```python
from build123d import *

# Parameters (mm, degrees)
SKETCH_1_R      = 63
SKETCH_1_R_2    = 1.25
EXTRUDE_1_DEPTH = 15
FILLET_1_R      = 3


with BuildPart() as part:
    # 草图1 → 凸台-拉伸1 (new body)
    with BuildSketch(Plane.XY):
        Circle(SKETCH_1_R)
        with Locations((0, 55)):
            Circle(SKETCH_1_R_2, mode=Mode.SUBTRACT)
        with Locations((47.631397208, 27.5)):
            Circle(SKETCH_1_R_2, mode=Mode.SUBTRACT)
        with Locations((47.631397208, -27.5)):
            Circle(SKETCH_1_R_2, mode=Mode.SUBTRACT)
        with Locations((0, -55)):
            Circle(SKETCH_1_R_2, mode=Mode.SUBTRACT)
        with Locations((-47.631397208, -27.5)):
            Circle(SKETCH_1_R_2, mode=Mode.SUBTRACT)
        with Locations((-47.631397208, 27.5)):
            Circle(SKETCH_1_R_2, mode=Mode.SUBTRACT)
        with BuildLine():
            Line((-2.5, 55), (-2.724459655, 59.938112413))
            ThreePointArc((-2.724459655, 59.938112413), (-30, 51.961524227), (-50.545698177, 32.328507479))
            Line((-50.545698177, 32.328507479), (-46.381397208, 29.665063509))
            ThreePointArc((-46.381397208, 29.665063509), (-45.466333699, 26.25), (-48.881397208, 25.334936491))
            Line((-48.881397208, 25.334936491), (-53.270157832, 27.609604933))
            ThreePointArc((-53.270157832, 27.609604933), (-60, 0), (-53.270157832, -27.609604933))
            Line((-53.270157832, -27.609604933), (-48.881397208, -25.334936491))
            ThreePointArc((-48.881397208, -25.334936491), (-45.466333699, -26.25), (-46.381397208, -29.665063509))
            Line((-46.381397208, -29.665063509), (-50.545698177, -32.328507479))
            ThreePointArc((-50.545698177, -32.328507479), (-30, -51.961524227), (-2.724459655, -59.938112413))
            Line((-2.724459655, -59.938112413), (-2.5, -55))
            ThreePointArc((-2.5, -55), (0, -52.5), (2.5, -55))
            Line((2.5, -55), (2.724459655, -59.938112413))
            ThreePointArc((2.724459655, -59.938112413), (30, -51.961524227), (50.545698177, -32.328507479))
            Line((50.545698177, -32.328507479), (46.381397208, -29.665063509))
            ThreePointArc((46.381397208, -29.665063509), (45.466333699, -26.25), (48.881397208, -25.334936491))
            Line((48.881397208, -25.334936491), (53.270157832, -27.609604933))
            ThreePointArc((53.270157832, -27.609604933), (60, 0), (53.270157832, 27.609604933))
            Line((53.270157832, 27.609604933), (48.881397208, 25.334936491))
            ThreePointArc((48.881397208, 25.334936491), (45.466333699, 26.25), (46.381397208, 29.665063509))
            Line((46.381397208, 29.665063509), (50.545698177, 32.328507479))
            ThreePointArc((50.545698177, 32.328507479), (30, 51.961524227), (2.724459655, 59.938112413))
            Line((2.724459655, 59.938112413), (2.5, 55))
            ThreePointArc((2.5, 55), (0, 52.5), (-2.5, 55))
        make_face(mode=Mode.SUBTRACT)
    extrude(amount=EXTRUDE_1_DEPTH)

    # 圆角1
    fillet_1_edges = [part.edges().sort_by_distance(p)[0] for p in [
        (-2.724459655, 59.938112413, 7.5),
        (-50.545698177, 32.328507479, 7.5),
        (-53.270157832, 27.609604933, 7.5),
        (-53.270157832, -27.609604933, 7.5),
        (-50.545698177, -32.328507479, 7.5),
        (-2.724459655, -59.938112413, 7.5),
        (2.724459655, -59.938112413, 7.5),
        (50.545698177, -32.328507479, 7.5),
        (53.270157832, -27.609604933, 7.5),
        (53.270157832, 27.609604933, 7.5),
        (50.545698177, 32.328507479, 7.5),
        (2.724459655, 59.938112413, 7.5),
    ]]
    fillet(fillet_1_edges, radius=FILLET_1_R)


solid = part.part
```
Model file for the job. Use its own axes, mm. Coordinates: 2 decimals unless noted, no trailing zeros. Order: outer loops, then holes, each group sorted by start corner. A loop starts at its lowest first (then second) coordinate and runs counter-clockwise, first axis right, second up. Notation, with made-up numbers: (38.5, 1) - (95.5, 1) arc R11 cw to (95.5, 15) - close; hole circle Ø10 at (56, -19.5). An arc over 180 degrees is marked (long way). Return JSON: item names as keys, results as strings. Group by question number.
1) Saw through at A-A, the plane y = 0. Write the cut outline in (x, z).
2) Probe line 1 (Y direction, x = 0, z = 6.5); line 2 (X direction, y = 30.5, z = 12); line 3 (Y direction, x = 46.5, z = 2). List the from-to ranges inside material, lowest first. Write a range as from..to.
3) Saw through at C-C, the plane z = 4.25. Count the separate pieces of the cut face and the enclosed holes in it, plus the area to 3 significant figures.
4) Mould opens along Y. For faces 1 (the cylindrical face through (-8.201, 62.464, 7.395)), 2 (the cylindrical face through (-49.288, 32.664, 7.605)), 3 (the cylindrical face through (29.69, -52.14, 7.4)), 4 (the flat face through (46, -28, 0)) say: released by +Y, released by -Y, zero draft, split by the parting line, or undercut.
5) Flat gauge pins, fed straight in: P1, Ø4, axis at x = 1, z = 11, coming from the +Y side; P2, Ø2, axis at y = 9.5, z = 12.5, coming from the -X side; P3, Ø8, axis at y = 38.5, z = 10.5, coming from the -X side. Where does each tip first touch, or does it go through?
6) Saw through at B-B, the plane x = -29.5. Write the cut outline in (y, z), plus the area to 3 significant figures.
Values found:
{
 "1": {"outline": "(-63, 0) - (-60, 0) - (-60, 15) - (-63, 15) - close; (60, 0) - (63, 0) - (63, 15) - (60, 15) - close"},
 "2": {"line 1": "y = -63..-56.25, -53.75..-52.5, 52.5..53.75, 56.25..63", "line 2": "x = -55.12..-47.69, 47.69..55.12", "line 3": "y = -42.51..-37.92, -29.74..-28.03, -26.97..-25.27, 25.27..26.97, 28.03..29.74, 37.92..42.51"},
 "3": {"separate pieces": "1", "enclosed holes": "7", "area": "1,370 mm²"},
 "4": {"face 1": "split by the parting line", "face 2": "undercut", "face 3": "undercut", "face 4": "zero draft"},
 "5": {"P1": "stops at y = 63", "P2": "stops at x = -62.42", "P3": "stops at x = -52.71"},
 "6": {"outline": "(-55.67, 0) - (-52.25, 0) - (-52.25, 15) - (-55.67, 15) - close; (52.25, 0) - (55.67, 0) - (55.67, 15) - (52.25, 15) - close", "area": "103 mm²"}
}
